The model under review builds one solid part; all positions refer to its coordinate system, in mm. A direction names the side the tool comes from. Round coordinates to 2 decimals unless told otherwise and drop trailing zeros. Order: outer loops, then holes, each group sorted by start corner. A loop starts at its lowest first (then second) coordinate and runs counter-clockwise, first axis right, second up. Notation, with made-up numbers: (36, 80) - (89, 80) arc R31 ccw to (89, 118) - close; hole circle Ø1 at (87, 2.25). An arc over 180 degrees is marked (long way). One line per question, with ' | ' between items. Start each with the question number.
Item 1: Add section B-B on z = 18. State the section outline as (x, y) points (3 decimals), and give its area (3 significant figures).
Item 2: For L1, parallel to X at y = 7, z = 100.5; L2, parallel to Z at x = -88.5, y = 16; L3, parallel to Z at x = 58, y = -3, list the stretches that pass through material, from the lowest coordinate up. Write a range as [from, to].
Item 3: Insertion check: pin 1 Ø1 at (x, y) = (-17, 7) entering from +Z; pin 2 Ø6.5 at (x, y) = (113.35, 8.62) entering from -Z; pin 3 Ø1.5 at (y, z) = (0, 20) entering from +X; pin 4 Ø1 at (y, z) = (7.5, 88) entering from +X. Each pin has a flat end and moves straight along its axis. Give the tip position at first contact, or say it passes through.
Item 4: Tool access review of faces 1 (the face through (-15, 15, 29)), 2 (the face through (-105, 0, 123)), 3 (the face through (-55.742, -0.21, 45.036)), 4 (the face through (68, 0, 30)), 5 (the face through (-100, 0, 87)): name each direction out of +Z, -Z, +X, -X, +Y, -Y from which nothing blocks a thin tool from reaching the whole face with its end or side.
Item 5: Draft analysis for pull direction X (two halves, no side actions). For faces 6 (the face through (-89.496, 0.198, 138.958)), 7 (the face through (-15, -15, 29)), 8 (the face through (100, -13, 15)), state which applies: +X half, -X half, draft (parallel to the pull), parting line (faces both ways), or undercut.
Item 6: Add section C-C on x = -85. State the section outline as (y, z) points, and give its area (3 significant figures).
Item 7: Add section D-D on y = 0. State the section outline as (x, z) points, and give its area (3 significant figures).
Item 8: Add section A-A on y = 24. State the section outline as (x, z) points, and give its area (3 significant figures).
from build123d import *

# Parameters (mm, degrees)
EXTRUDE_1_DEPTH          = 30
SKETCH_12_W              = 30
SKETCH_12_H              = 93
EXTRUDE_6_DEPTH          = 30
SKETCH_16_R              = 30
EXTRUDE_9_DEPTH          = 13
FILLET_1_R               = 50
FILLET_2_R               = 50
SKETCH_17_R              = 2
CUT_EXTRUDE_1_DEPTH      = 193.846857699
PATTERN_CIRCULAR_1_COUNT = 6
SKETCH_18_R              = 4.5
EXTRUDE_10_DEPTH         = 6


with BuildPart() as part:
    # 草图1 → 凸台-拉伸1 (new body)
    with BuildSketch(Plane.XY):
        Polygon((100, -10), (100, 0), (100, 10), (100, 15), (-100, 15), (-100, -15), (100, -15), align=None)
        with BuildLine():
            Line((100, 10), (100, 0))
            Line((100, 0), (100, -10))
            ThreePointArc((100, -10), (158.284271247, 0), (100, 10))
        make_face()
    extrude(amount=EXTRUDE_1_DEPTH)

    # 草图12 → 凸台-拉伸6 (add)
    with BuildSketch(Plane(origin=(0, 15, 0), x_dir=(1, 0, 0), z_dir=(0, 1, 0))):
        with Locations((-85, -76.5)):
            Rectangle(SKETCH_12_W, SKETCH_12_H)
    extrude(amount=-EXTRUDE_6_DEPTH)

    # 草图16 → 凸台-拉伸9 (add)
    with BuildSketch(Plane.XY.offset(123)):
        with Locations(Location((-85, 0, 0), (0, 0, 180))):
            Circle(SKETCH_16_R)
    extrude(amount=EXTRUDE_9_DEPTH)

    # 圆角1
    fillet_1_edges = [part.edges().sort_by_distance(p)[0] for p in [
        (-70, 0, 30),
    ]]
    fillet(fillet_1_edges, radius=FILLET_1_R)

    # 圆角2
    fillet_2_edges = [part.edges().sort_by_distance(p)[0] for p in [
        (-100, 0, 0),
    ]]
    fillet(fillet_2_edges, radius=FILLET_2_R)

    # 草图17 → 切除-拉伸1 (cut, through all)
    with BuildSketch(Plane.XY.offset(30)):
        with Locations((128.284271247, 17.25)):
            Circle(SKETCH_17_R)
    cut_extrude_1 = extrude(amount=-CUT_EXTRUDE_1_DEPTH, mode=Mode.SUBTRACT)

    # 阵列(圆周)1: 切除-拉伸1 ×6 about axis
    pattern_circular_1_axis = Axis((128.284271247, 0, 0), (0, 0, 1))
    for i in range(1, PATTERN_CIRCULAR_1_COUNT):
        add(cut_extrude_1.rotate(pattern_circular_1_axis, i * 360 / PATTERN_CIRCULAR_1_COUNT), mode=Mode.SUBTRACT)

    # 草图18 → 凸台-拉伸10 (add)
    with BuildSketch(Plane.XY.offset(136)):
        with Locations((-85, 0)):
            Circle(SKETCH_18_R)
    extrude(amount=EXTRUDE_10_DEPTH)


solid = part.part
Determined:
1) outline: (-88.419, -15) - (100, -15) - (100, -10) arc R30 ccw (long way) to (100, 10) - (100, 15) - (-88.419, 15) - close; hole circle Ø4 at (113.345, -8.625); hole circle Ø4 at (113.345, 8.625); hole circle Ø4 at (128.284, -17.25); hole circle Ø4 at (128.284, 17.25); hole circle Ø4 at (143.223, -8.625); hole circle Ø4 at (143.223, 8.625) | area: 8,380 mm2
2) L1: [-100, -70] | L2: [123, 136] | L3: [0, 30]
3) pin 1: z = 30 | pin 2: z = 0 | pin 3: x = 158.28 | pin 4: x = -70
4) face 1: -Z, -X, +Y | face 2: none | face 3: +X, +Y, -Y | face 4: +Z, +X, +Y, -Y | face 5: -Z, -X, +Y, -Y
5) face 6: parting line | face 7: draft | face 8: undercut
6) outline: (-30, 123) - (-15, 123) - (-15, 14.29) - (15, 14.29) - (15, 123) - (30, 123) - (30, 136) - (4.5, 136) - (4.5, 142) - (-4.5, 142) - (-4.5, 136) - (-30, 136) - close | area: 4,100 mm2
7) outline: (-115, 123) - (-100, 123) - (-100, 50) arc R50 ccw to (-50, 0) - (158.28, 0) - (158.28, 30) - (-20, 30) arc R50 cw to (-70, 80) - (-70, 123) - (-55, 123) - (-55, 136) - (-80.5, 136) - (-80.5, 142) - (-89.5, 142) - (-89.5, 136) - (-115, 136) - close | area: 11,400 mm2
8) outline: (-103, 123) - (-67, 123) - (-67, 136) - (-103, 136) - close; (110.28, 0) - (146.28, 0) - (146.28, 30) - (110.28, 30) - close | area: 1,550 mm2
